Source: three-view drawing plus pictorial views. Frame: mm from the lowest corner of the part. A direction names the side the tool comes from. Round coordinates to 2 decimals unless told otherwise and drop trailing zeros. Write each loop counter-clockwise with the first axis right and the second up, starting at its lowest first coordinate (ties: lowest second). Pieces come first, ordered by that corner, then holes. Notation, with made-up numbers: M -15,-9 L 43,-9 A20 cw 43,10 Z; hole C -37.75,-16 d7. An arc over 180 degrees is marked long. Answer in a Markdown table with one row per item.
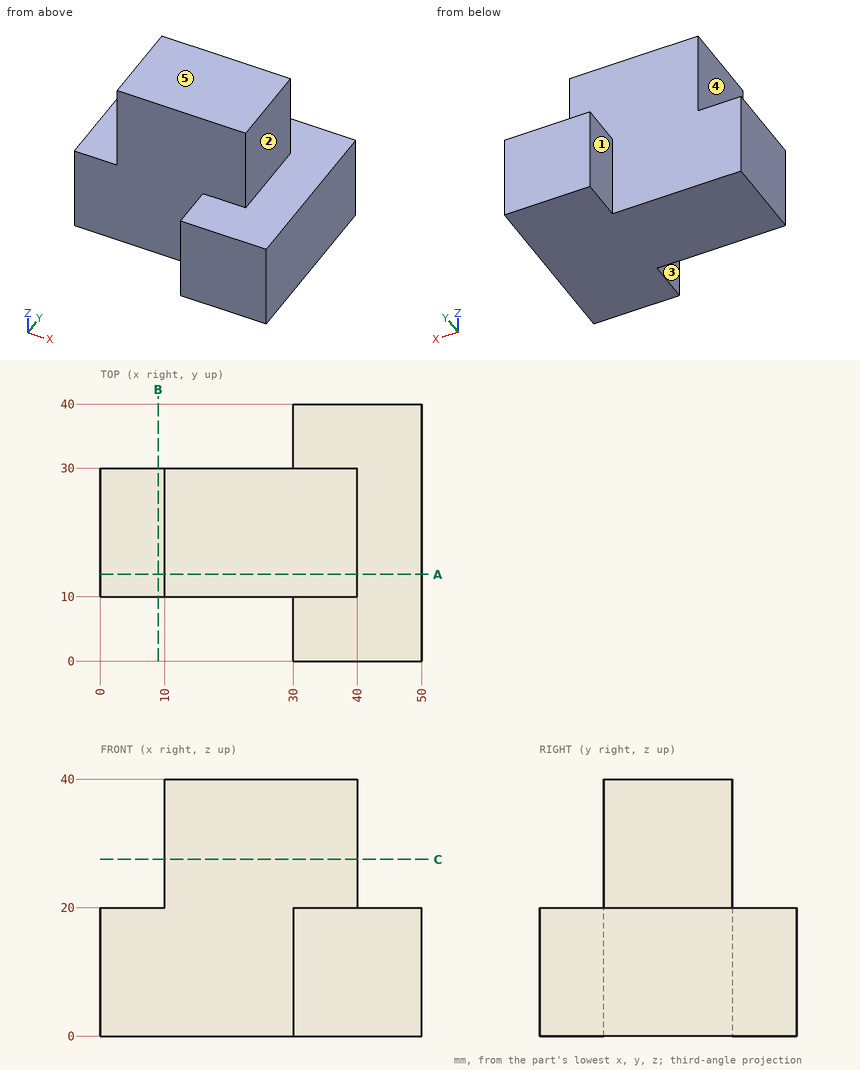
Q1. Section A-A (y = 13.5). Return loops of the section in (x, z).
Solutions:
| item | result |
|---|---|
| outline | M 0,0 L 50,0 L 50,20 L 40,20 L 40,40 L 10,40 L 10,20 L 0,20 Z |
Q2. Access query for the marked faces 1, 2, 3, 4 and 5. Directions: +Z, -Z, +X, -X, +Y, -Y. A direction counts if a zero-diameter tool reaches every point of the face in a straight line with its end or side. Return the directions, or none.
Solutions:
| item | result |
|---|---|
| face 1 | +Z, -Z, -X, +Y |
| face 2 | +Z, +X, +Y, -Y |
| face 3 | +Z, -Z, -X, -Y |
| face 4 | +Z, -X, +Y, -Y |
| face 5 | +Z, +X, -X, +Y, -Y |
Q3. Section B-B (x = 9). Return loops of the section in (y, z), and give its area (3 significant figures).
Solutions:
| item | result |
|---|---|
| outline | M 10,0 L 30,0 L 30,20 L 10,20 Z |
| area | 400 mm2 |
Q4. Section C-C (z = 27.5). Return loops of the section in (x, y).
Solutions:
| item | result |
|---|---|
| outline | M 10,10 L 40,10 L 40,30 L 10,30 Z |
Q5. Contact query for flat-ended pins moving along their axis: pin 1 Ø12 at (y, z) = (13.5, 29) entering from +X; pin 2 Ø3 at (x, y) = (24.5, 33) entering from -Z; pin 3 Ø11 at (y, z) = (3, 11) entering from -X; pin 4 Ø20 at (x, z) = (15.5, 12) entering from +Y. Output: stop coordinate, or through.
Solutions:
| item | result |
|---|---|
| pin 1 | stops at x = 40 |
| pin 2 | passes through |
| pin 3 | stops at x = 30 |
| pin 4 | stops at y = 30 |
Q6. Material intervals for probe 1 along X at (y, z) = (16, 32); probe 2 along Y at (x, z) = (12, 37.5); probe 3 along X at (y, z) = (5.5, 9), sorted ascending.
Solutions:
| item | result |
|---|---|
| probe 1 | x = 10 to 40 |
| probe 2 | y = 10 to 30 |
| probe 3 | x = 30 to 50 |
